Here's how the part is built. I have some questions about the finished solid (model axes, mm). Face numbers are marked on the shaded views. Give positions to 0.01 mm unless a question says otherwise; leave off trailing zeros. Write each loop counter-clockwise with the first axis right and the second up, starting at its lowest first coordinate (ties: lowest second). Pieces come first, ordered by that corner, then holes. Notation, with made-up numbers: (-0.75, -12) -> (15.25, -12) arc R8 ccw to (15.25, -2) -> close; hole circle Ø2 at (33.5, 32). An arc over 180 degrees is marked (long way). Return JSON: item names as keys, results as strings.
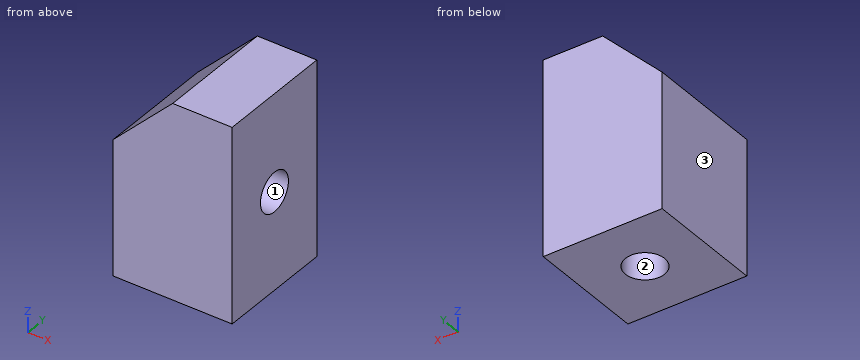
from build123d import *

# Parameters (mm, degrees)
SKETCH1_W                 = 10
SKETCH1_H                 = 16.35
BOSS_EXTRUDE1_DEPTH       = 10
CHAMFER1_SIZE             = 5
M4X0_7_TAPPED_HOLE1_D     = 3.3
M4X0_7_TAPPED_HOLE1_DEPTH = 4.825
M4X0_7_TAPPED_HOLE1_TIP   = 0.991420021
M4X0_7_TAPPED_HOLE2_D     = 3.3
M4X0_7_TAPPED_HOLE2_DEPTH = 4.825
M4X0_7_TAPPED_HOLE2_TIP   = 0.991420021


with BuildPart() as part:
    # Sketch1 → Boss-Extrude1 (new body)
    with BuildSketch(Plane(origin=(0, 0, 0), x_dir=(1, 0, 0), z_dir=(0, 1, 0))):
        Rectangle(SKETCH1_W, SKETCH1_H)
    extrude(amount=BOSS_EXTRUDE1_DEPTH)

    # Chamfer1
    chamfer1_edges = [part.edges().sort_by_distance(p)[0] for p in [
        (-5, 5, 8.175),
    ]]
    chamfer(chamfer1_edges, length=CHAMFER1_SIZE)

    # M4x0.7 Tapped Hole1
    with Locations(Plane(origin=(5, 0, 0), x_dir=(0, 0, -1), z_dir=(1, 0, 0))):
        with Locations((0, 5)):
            Hole(M4X0_7_TAPPED_HOLE1_D / 2, depth=M4X0_7_TAPPED_HOLE1_DEPTH)
            with Locations((0, 0, -(M4X0_7_TAPPED_HOLE1_DEPTH + M4X0_7_TAPPED_HOLE1_TIP / 2))):  # 118° drill point
                Cone(0, M4X0_7_TAPPED_HOLE1_D / 2, M4X0_7_TAPPED_HOLE1_TIP, mode=Mode.SUBTRACT)

    # M4x0.7 Tapped Hole2
    with Locations(Plane(origin=(0, 0, -8.175), x_dir=(-1, 0, 0), z_dir=(0, 0, -1))):
        with Locations((0, 5)):
            Hole(M4X0_7_TAPPED_HOLE2_D / 2, depth=M4X0_7_TAPPED_HOLE2_DEPTH)
            with Locations((0, 0, -(M4X0_7_TAPPED_HOLE2_DEPTH + M4X0_7_TAPPED_HOLE2_TIP / 2))):  # 118° drill point
                Cone(0, M4X0_7_TAPPED_HOLE2_D / 2, M4X0_7_TAPPED_HOLE2_TIP, mode=Mode.SUBTRACT)


solid = part.part
1. Suppose I cut it at C-C, the plane z = 7.25. List the corners of the cut face in (x, y) for me (3 decimals), and give its area (4 significant figures).
Taken from the geometry:
{"outline": "(-0.925, 0) -> (5, 0) -> (5, 10) -> (-0.925, 10) -> close", "area": "59.25 mm²"}
2. Suppose I cut it at A-A, the plane x = 4.5. List the corners of the cut face in (y, z) for me (3 decimals).
Taken from the geometry:
{"outline": "(0, -8.175) -> (10, -8.175) -> (10, 8.175) -> (0, 8.175) -> close; hole circle Ø3.3 at (5, 0)"}
3. If I drill on line 1 (Y direction, x = 0, z = -6.65); line 2 (X direction, y = 5, z = -6.25); line 3 (Z direction, x = 3.55, y = 5) (3 decimals), over which ranges is the centre line in solid material (lowest first)? Write a range as [from, to].
Taken from the geometry:
{"line 1": "y = [0, 3.35], [6.65, 10]", "line 2": "x = [-5, -1.65], [1.65, 5]", "line 3": "z = [-8.175, -1.65], [1.65, 8.175]"}
4. Suppose I cut it at B-B, the plane y = 2.75. List the corners of the cut face in (x, z) for me (3 decimals).
Taken from the geometry:
{"outline": "(-5, -8.175) -> (5, -8.175) -> (5, 8.175) -> (0, 8.175) -> (-5, 3.175) -> close"}
5. For pin 1 Ø1 at (x, y) = (-2, 4.5) entering from +Z (3 decimals), with a flat end and sliding along its axis, tell me the tip position at first contact or that it passes through.
Taken from the geometry:
{"pin 1": "stops at z = 6.675"}
6. Suppose I cut it at D-D, the plane x = -3.75. List the corners of the cut face in (y, z) for me (3 decimals).
Taken from the geometry:
{"outline": "(0, -8.175) -> (10, -8.175) -> (10, 4.425) -> (0, 4.425) -> close"}
7. If we mould it in two halves opening along X, with no side actions, what happens to the marked faces 1, 2 and 3? For each: released by +X, released by -X, zero draft, split by the parting line, or undercut.
Taken from the geometry:
{"face 1": "zero draft", "face 2": "undercut", "face 3": "released by -X"}
